from build123d import *

# Parameters (mm, degrees)
LOFT1_DEPTH             = 30
LOFT1_DRAFT             = 1.9091524
CUT_EXTRUDE2_DEPTH      = 33.499999989
CUT_EXTRUDE2_DEPTH_BACK = 33.499999989
FILLET5_R               = 1
SKETCH4_R               = 3
BOSS_EXTRUDE1_DEPTH     = 1.5
CUT_EXTRUDE3_START      = 3
SKETCH5_R               = 3
CUT_EXTRUDE3_DEPTH      = 3
SKETCH7_R               = 3
CUT_EXTRUDE5_DEPTH      = 1.5
BOSS_EXTRUDE2_START     = -3
SKETCH8_R               = 3
BOSS_EXTRUDE2_DEPTH     = 3
CUT_EXTRUDE6_DEPTH      = 23.235565384
CUT_EXTRUDE6_DEPTH_BACK = 23.235565384
CUT_EXTRUDE7_DEPTH      = 23.523598989
CUT_EXTRUDE7_DEPTH_BACK = 23.523598989
CUT_EXTRUDE8_DEPTH      = 36.642580329
CUT_EXTRUDE8_DEPTH_BACK = 36.642580329
SKETCH11_R              = 1.45


# Read off the part's stored shape, not the designer's step: Loft1
with BuildPart() as part:
    # Loft1 outline → Loft1 (with draft: the straight prism first)
    with BuildSketch(Plane(origin=(0, 30, 0), x_dir=(1, 0, 0), z_dir=(0, 1, 0))):
        Polygon((2.085786438, 6.5), (-2.085786438, 6.5), (-8.585786438, 0), (-2.085786438, -6.5), (2.085786438, -6.5), (8.585786438, 0), align=None)
    extrude(amount=-LOFT1_DEPTH)
    # Loft1: the draft: its side faces are tilted about the plane it starts from
    loft1_sides = [part.faces().sort_by_distance(p)[0] for p in [
        (0, 15, -6.5),
        (-5.335786438, 15, -3.25),
        (-5.335786438, 15, 3.25),
        (0, 15, 6.5),
        (5.335786438, 15, 3.25),
        (5.335786438, 15, -3.25),
    ]]
    draft(loft1_sides, Plane(origin=(0, 30, 0), x_dir=(1, 0, 0), z_dir=(0, 1, 0)), LOFT1_DRAFT)

    # Sketch3 → Cut-Extrude2 (cut, two sides: drawn at the far end of the back side and taken through both)
    with BuildSketch(Plane(origin=(0, 0, 0), x_dir=(0, 0, -1), z_dir=(1, 0, 0)).offset(-CUT_EXTRUDE2_DEPTH_BACK)):
        Polygon((0, 30), (0, 29), (-6.75862069, 22.24137931), (-6.5, 30), align=None)
        Polygon((0, 0), (0, 1), (-7.225806452, 8.225806452), (-7.5, 0), align=None)
    extrude(amount=CUT_EXTRUDE2_DEPTH + CUT_EXTRUDE2_DEPTH_BACK, mode=Mode.SUBTRACT)

    # Fillet5
    # the kernel refuses this fillet: 1 mm, written as the material it takes off along each edge
    with BuildSketch(Plane(origin=(8.515337072, 31.494456763, 0), x_dir=(-0.7059303394201505, -0.033277874761044414, -0.7074990734534847), z_dir=(0.04708816012216718, -0.9988907373563483, 0))) as fillet5_piece_1:
        with BuildLine():
            CenterArc((FILLET5_R * 0.998890737356, -FILLET5_R), FILLET5_R, 90, 89.936408669)
            Line((-FILLET5_R * 0.00110864672901, -FILLET5_R * 0.998890122125), (0, 0))
            Line((0, 0), (FILLET5_R * 0.998890737356, 0))
        make_face()
    extrude(amount=33.025547532, mode=Mode.SUBTRACT)
    with BuildSketch(Plane(origin=(-8.515337072, 31.494456763, 0), x_dir=(0.7059303394201496, -0.03327787476104438, -0.7074990734534856), z_dir=(-0.04708816012216718, -0.9988907373563483, 0))) as fillet5_piece_2:
        with BuildLine():
            CenterArc((FILLET5_R * 0.998890737356, FILLET5_R), FILLET5_R, 180.063591331, 89.936408669)
            Line((-FILLET5_R * 0.00110864672902, FILLET5_R * 0.998890122125), (0, 0))
            Line((0, 0), (FILLET5_R * 0.998890737356, 0))
        make_face()
    extrude(amount=33.025547532, mode=Mode.SUBTRACT)

    # Sketch4 → Boss-Extrude1 (add, symmetric)
    with BuildSketch(Plane(origin=(0, 0, 0), x_dir=(0, 0, -1), z_dir=(1, 0, 0))):
        with Locations((0, 30.5)):
            Circle(SKETCH4_R)
    extrude(amount=BOSS_EXTRUDE1_DEPTH, both=True)

    # Sketch5 → Cut-Extrude3 (cut)
    with BuildSketch(Plane(origin=(1.5, 0, 0), x_dir=(0, 0, -1), z_dir=(1, 0, 0)).offset(CUT_EXTRUDE3_START)):
        with Locations((0, 30.5)):
            Circle(SKETCH5_R)
    cut_extrude3 = extrude(amount=-CUT_EXTRUDE3_DEPTH, mode=Mode.SUBTRACT)

    # Mirror1: Cut-Extrude3 across plane
    add(cut_extrude3.mirror(Plane(origin=(0, 0, 0), x_dir=(0, 0, 1), z_dir=(1, 0, 0))), mode=Mode.SUBTRACT)

    # Sketch7 → Cut-Extrude5 (cut, symmetric)
    with BuildSketch(Plane(origin=(0, 0, 0), x_dir=(0, 0, -1), z_dir=(1, 0, 0))):
        with Locations((0, -0.5)):
            Circle(SKETCH7_R)
    extrude(amount=CUT_EXTRUDE5_DEPTH, both=True, mode=Mode.SUBTRACT)

    # Sketch8 → Boss-Extrude2 (add)
    with BuildSketch(Plane.ZY.offset(-1.5).offset(BOSS_EXTRUDE2_START)):
        with Locations((0, -0.5)):
            Circle(SKETCH8_R)
    boss_extrude2 = extrude(amount=BOSS_EXTRUDE2_DEPTH)

    # Mirror2: Boss-Extrude2 across plane
    add(boss_extrude2.mirror(Plane(origin=(0, 0, 0), x_dir=(0, 0, 1), z_dir=(1, 0, 0))))

    # Sketch9 → Cut-Extrude6 (cut, two sides: drawn at the far end of the back side and taken through both)
    with BuildSketch(Plane(origin=(0, 14.98387035, -0.499462345), x_dir=(1, 0, 0), z_dir=(0, 0.9994449069791544, -0.03331483023263851)).offset(-CUT_EXTRUDE6_DEPTH_BACK)):
        Polygon((-1, -4.495836802), (1, -4.495836802), (1, -5.495836802), (0, -6.495836802), (-1, -5.495836802), align=None)
    extrude(amount=CUT_EXTRUDE6_DEPTH + CUT_EXTRUDE6_DEPTH_BACK, mode=Mode.SUBTRACT)

    # Sketch10 → Cut-Extrude7 (cut, two sides: drawn at the far end of the back side and taken through both)
    with BuildSketch(Plane(origin=(0, 14.750277469, 0.491675916), x_dir=(1, 0, 0), z_dir=(0, 0.9994449069791544, 0.03331483023263851)).offset(-CUT_EXTRUDE7_DEPTH_BACK)):
        Polygon((-1, 6.495836802), (1, 6.495836802), (1, 5.495836802), (0, 4.495836802), (-1, 5.495836802), align=None)
    extrude(amount=CUT_EXTRUDE7_DEPTH + CUT_EXTRUDE7_DEPTH_BACK, mode=Mode.SUBTRACT)

    # Sketch11 → Cut-Extrude8 (cut, two sides: drawn at the far end of the back side and taken through both)
    with BuildSketch(Plane(origin=(0, 0, 0), x_dir=(0, 0, -1), z_dir=(1, 0, 0)).offset(-CUT_EXTRUDE8_DEPTH_BACK)):
        with Locations((0, 30.5)):
            Circle(SKETCH11_R)
        with Locations((0, -0.5)):
            Circle(SKETCH11_R)
    extrude(amount=CUT_EXTRUDE8_DEPTH + CUT_EXTRUDE8_DEPTH_BACK, mode=Mode.SUBTRACT)


solid = part.part
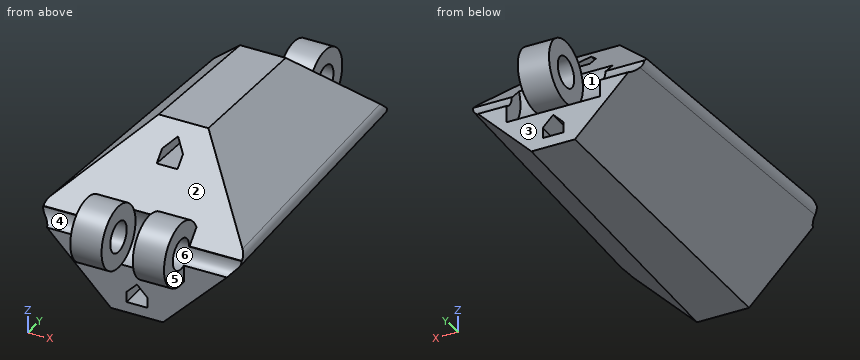
Build history of the part. All positions in model axes, mm. Face numbers are marked on the shaded views. A direction names the side the tool comes from. Round coordinates to 2 decimals unless told otherwise and drop trailing zeros. Write each loop counter-clockwise with the first axis right and the second up, starting at its lowest first coordinate (ties: lowest second). Pieces come first, ordered by that corner, then holes. Notation, with made-up numbers: M 39.25,28.25 L 62.25,28.25 A23 cw 62.25,53.25 Z; hole C 16.25,21.5 d1. An arc over 180 degrees is marked long. Answer in a Markdown table with one row per item.
1. Flat gauge pins, fed straight in: P1, Ø2, axis at y = 8.5, z = -6, coming from the -X side; P2, Ø0.5, axis at y = 16, z = 4, coming from the -X side; P3, Ø1.2, axis at y = 28, z = 0, coming from the +X side. Where does each tip first touch, or does it go through?
Geometry check:
| item | result |
|---|---|
| P1 | x = -4.6 |
| P2 | x = -5.5 |
| P3 | x = 8.29 |
2. Mould opens along Z. For the marked faces 1, 2, 3 and 4 say: +Z half, -Z half, draft (parallel to the pull), parting line (faces both ways), or undercut.
Geometry check:
| item | result |
|---|---|
| face 1 | undercut |
| face 2 | +Z half |
| face 3 | draft |
| face 4 | undercut |
3. Saw through at A-A (y = 30.5). List the corners of the cut face in (x, z), and give its area (3 significant figures).
Geometry check:
| item | result |
|---|---|
| outline | M -1.5,-3 L 1.5,-3 L 1.5,-1.45 L -1.5,-1.45 Z; M -1.5,1.45 L 1.5,1.45 L 1.5,3 L -1.5,3 Z |
| area | 9.30 mm2 |
4. Saw through at B-B (y = -0.5). List the corners of the cut face in (x, z), and give its area (3 significant figures).
Geometry check:
| item | result |
|---|---|
| outline | M -4.5,-3 L -1.5,-3 L -1.5,-1.45 L -4.5,-1.45 Z; M -4.5,1.45 L -1.5,1.45 L -1.5,3 L -4.5,3 Z; M 1.5,-3 L 4.5,-3 L 4.5,-1.45 L 1.5,-1.45 Z; M 1.5,1.45 L 4.5,1.45 L 4.5,3 L 1.5,3 Z |
| area | 18.6 mm2 |
5. Saw through at C-C (z = 2.25). List the corners of the cut face in (x, y), and give its area (3 significant figures).
Geometry check:
| item | result |
|---|---|
| outline | M -7.6,3.25 L 7.6,3.25 L 6.49,26.75 L -6.49,26.75 Z; M -4.5,-2.48 L -1.5,-2.48 L -1.5,1.48 L -4.5,1.48 Z; M -1.5,28.52 L 1.5,28.52 L 1.5,32.48 L -1.5,32.48 Z; M 1.5,-2.48 L 4.5,-2.48 L 4.5,1.48 L 1.5,1.48 Z |
| area | 367 mm2 |
6. Saw through at D-D (x = 5). List the corners of the cut face in (y, z).
Geometry check:
| item | result |
|---|---|
| outline | M 0,-5 L 30,-3.59 L 30,-1.36 A1.45 cw 29.05,0 L 29,0 L 25.19,3.81 L 5.73,4.73 L 1,0 L 0.95,0 A1.45 cw 0,-1.36 Z |
7. Probe L1, parallel to Y at x = 3.75, z = 0; L2, parallel to Z at x = 0.5, y = 30.5; L3, parallel to Y at x = -6.25, z = 0. List the from-to ranges inside material, lowest first. Write a range as [from, to].
Geometry check:
| item | result |
|---|---|
| L1 | [-3.5, -1.95], [0.95, 27.5] |
| L2 | [-3, -1.45], [1.45, 3] |
| L3 | [1, 29] |
8. Which spindle directions (+Z, -Z, +X, -X, +Y, -Y) get a long thin tool onto all of the face, cutting with end or side? Do the marked faces 5 and 6. Say none if no direction does.
Geometry check:
| item | result |
|---|---|
| face 5 | +Z, +X, -Y |
| face 6 | +X, -X |
